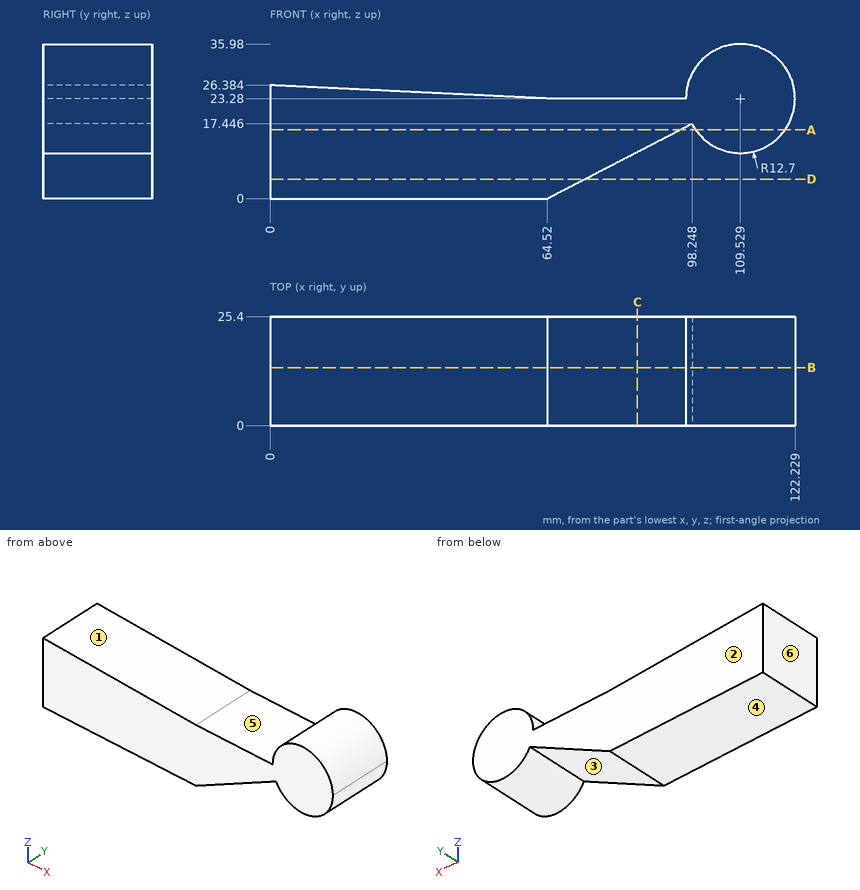
The figure shows three views and two pictorial views of one solid part (mm, origin at its lowest corner). Answer the questions. A direction names the side the tool comes from. Give positions to 0.01 mm unless a question says otherwise; leave off trailing zeros. Write each loop counter-clockwise with the first axis right and the second up, starting at its lowest first coordinate (ties: lowest second). Pieces come first, ordered by that corner, then holes. Notation, with made-up numbers: M 4.25,52.5 L 22.25,52.5 A30 cw 22.25,89.5 Z; hole C 42,-33 d9. An arc over 180 degrees is marked long. One line per item, written item: value. Start each with the question number.
(1) Find section A-A (z = 16). Determine the outline of the cut face in (x, y) (1 decimal).
(2) A tool of negligible diameter and unlimited length cuts with its end or side. For the marked faces 1, 2 and 3, from which of +Z, -Z, +X, -X, +Y, -Y can it reach the whole face along a straight path? Write none if from no direction.
(3) Find section C-C (x = 85.5). Determine the outline of the cut face in (y, z), plus the area to 3 significant figures.
(4) Find section B-B (y = 13.5). Determine the outline of the cut face in (x, z) (1 decimal), plus the area to 3 significant figures.
(5) Determine the mould class of the marked faces 4, 5 and 6 for opening direction X: pulls with the +X half, pulls with the -X half, needs draft (parallel to the pull), parting line crosses it, or undercut.
(6) Find the intervals of material crossed by line 1 (X direction, y = 15.5, z = 17) (1 decimal); line 2 (X direction, y = 22.5, z = 12.5) (1 decimal); line 3 (Z direction, x = 68.5, y = 22), in increasing order.
(7) Find section D-D (z = 4.5). Determine the outline of the cut face in (x, y).
(8) Flat-ended cylindrical pins translate along their axes: pin 1 Ø12 at (x, y) = (49.5, 11.5) entering from +Z; pin 2 Ø12.5 at (x, y) = (87, 17.5) entering from +Z; pin 3 Ø10 at (x, y) = (91.5, 3) entering from -Z. Find the tip coordinate at first contact, or state that the pin passes through.
Results below:
1. outline: M 0,0 L 95.5,0 L 95.5,25.4 L 0,25.4 Z; M 99.1,0 L 119.9,0 L 119.9,25.4 L 99.1,25.4 Z
2. face 1: +Z, +Y, -Y
2. face 2: +Z, -Z, +X, -X, +Y
2. face 3: -Z, +Y, -Y
3. outline: M 0,10.85 L 25.4,10.85 L 25.4,23.28 L 0,23.28 Z
3. area: 316 mm^2
4. outline: M 0,0 L 64.5,0 L 98.2,17.4 A12.7 ccw long 96.8,23.3 L 64.5,23.3 L 0,26.4 Z
4. area: 2,590 mm^2
5. face 4: needs draft
5. face 5: undercut
5. face 6: pulls with the -X half
6. line 1: x = 0 to 97.4, 98.5 to 120.6
6. line 2: x = 0 to 88.7, 102.8 to 116.2
6. line 3: z = 2.06 to 23.28
7. outline: M 0,0 L 73.22,0 L 73.22,25.4 L 0,25.4 Z
8. pin 1: stops at z = 24.29
8. pin 2: stops at z = 23.28
8. pin 3: stops at z = 11.37
